The model under review builds one solid part; all positions refer to its coordinate system, in mm. A direction names the side the tool comes from. Coordinates: 2 decimals unless noted, no trailing zeros. Order: outer loops, then holes, each group sorted by start corner. A loop starts at its lowest first (then second) coordinate and runs counter-clockwise, first axis right, second up. Notation, with made-up numbers: M -33,-40 L -29,-40 A30 ccw -29,-13 Z; hole C 4,54.25 d5. An arc over 180 degrees is marked long. Write each question's results on one line, items separated by ' | '.
from build123d import *

# Parameters (mm, degrees)
F1_R     = 32.7
F1_R_2   = 5
F2_DEPTH = 1.8
F0_R     = 32.7
F3_DEPTH = 46.6
F4_R     = 2.65
F5_DEPTH = 44.601471
F6_R     = 5.5
F7_DEPTH = 39.6


with BuildPart() as f2:
    # F1 (on Front) → F2 (new body)
    with BuildSketch(Plane.XZ):
        Circle(F1_R)
        Circle(F1_R_2, mode=Mode.SUBTRACT)
    extrude(amount=F2_DEPTH)

    # F0 (on Front) → F3 (join)
    with BuildSketch(Plane.XZ):
        with BuildLine():
            ThreePointArc((32.077406, -10), (33.217171, -5.057625), (33.6, 0))
            ThreePointArc((33.6, 0), (33.217171, 5.057625), (32.077406, 10))
            ThreePointArc((32.077406, 10), (-33.6, 0), (32.077406, -10))
        make_face()
        Circle(F0_R, mode=Mode.SUBTRACT)
        with BuildLine():
            Line((42.851, 0), (33.6, 0))
            ThreePointArc((33.6, 0), (33.217171, -5.057625), (32.077406, -10))
            Line((32.077406, -10), (42.851, -10))
            Line((42.851, -10), (42.851, -4.75))
            Line((42.851, -4.75), (42.851, 0))
        make_face()
        with BuildLine():
            ThreePointArc((32.077406, 10), (33.217171, 5.057625), (33.6, 0))
            Line((33.6, 0), (42.851, 0))
            Line((42.851, 0), (42.851, 4.75))
            Line((42.851, 4.75), (42.851, 10))
            Line((42.851, 10), (32.077406, 10))
        make_face()
        Polygon((42.851, 4.75), (42.851, 0), (42.851, -4.75), (44.600471, -3), (44.600471, 3), align=None)
    extrude(amount=F3_DEPTH)

    # F4 (on Right) → F5 (cut, through all)
    with BuildSketch(Plane.YZ):
        with Locations((-11.8, 0)):
            Circle(F4_R)
        with Locations((-36.6, 0)):
            Circle(F4_R)
    extrude(amount=F5_DEPTH, mode=Mode.SUBTRACT)

    # F6 (on Right) → F7 (cut)
    with BuildSketch(Plane.YZ):
        with Locations((-11.8, 0)):
            Circle(F6_R)
        with Locations((-36.6, 0)):
            Circle(F6_R)
    extrude(amount=F7_DEPTH, mode=Mode.SUBTRACT)


solid = f2.part
1) For pin 1 (5 mm diameter, centred on y = -13, z = -7.5, fed in from -X); pin 2 (2 mm diameter, centred on x = 23, z = 11.5, fed in from -Y); pin 3 (8.5 mm diameter, centred on x = 38, y = -12.5, fed in from -Z); pin 4 (8 mm diameter, centred on x = 0, z = 0, fed in from -Y), all flat-tipped, find the tip position at first contact; note any pin that passes through.
Solutions:
pin 1: x = -33.23 | pin 2: y = -1.8 | pin 3: z = -10 | pin 4: through
2) Take a section at C-C on y = -22. State the section outline as (x, z) points, plus the area to 3 significant figures.
Solutions:
outline: M 32.08,-10 L 42.85,-10 L 42.85,-4.75 L 44.6,-3 L 44.6,3 L 42.85,4.75 L 42.85,10 L 32.08,10 A33.6 ccw long Z; hole C 0,0 d65.4 | area: 396 mm2
3) The part is to be moulded in two halves that separate along Z. For faces 6 (the cylindrical face through (-33.573, -22.974, 1.335)), 7 (the cylindrical face through (35.866, -17.295, 0.242)), 8 (the flat face through (37, -23, -10)), say which applies: pulls with the +Z half, pulls with the -Z half, needs draft (parallel to the pull), parting line crosses it, or undercut.
Solutions:
face 6: parting line crosses it | face 7: undercut | face 8: pulls with the -Z half
4) To check wall thickness, follow line 1 along Y through (x, z) = (42.8, 0); line 2 along Y through (x, z) = (35, 0); line 3 along Z through (x, y) = (0, -31). State the ranges of each line that lie inside material, in increasing order.
Solutions:
line 1: -46.6 to -39.25, -33.95 to -14.45, -9.15 to 0 | line 2: -46.6 to -42.1, -31.1 to -17.3, -6.3 to 0 | line 3: -33.6 to -32.7, 32.7 to 33.6
5) For faces 1 (the flat face through (7, -1.8, 0)), 2 (the cylindrical face through (42.065, -39.247, 0.117)), 3 (the flat face through (42.851, -23, -7)), 4 (the flat face through (42.851, -23, 7)), 5 (the flat face through (39.6, -35, 3)), list the 3-axis set-ups (+Z, -Z, +X, -X, +Y, -Y) from which the entire face can be reached by the end or side of a thin tool; tool diameter is ignored.
Solutions:
face 1: -Y | face 2: +X | face 3: -Z, +X, +Y, -Y | face 4: +Z, +X, +Y, -Y | face 5: none
6) Take a section at A-A on x = 0. State the section outline as (y, z) points, plus the area to 3 significant figures.
Solutions:
outline: M -46.6,-33.6 L 0,-33.6 L 0,-5 L -1.8,-5 L -1.8,-32.7 L -46.6,-32.7 Z; M -46.6,32.7 L -1.8,32.7 L -1.8,5 L 0,5 L 0,33.6 L -46.6,33.6 Z | area: 184 mm2
7) Take a section at B-B on z = 0. State the section outline as (x, y) points, plus the area to 3 significant figures.
Solutions:
outline: M -33.6,-46.6 L -32.7,-46.6 L -32.7,-1.8 L -5,-1.8 L -5,0 L -33.6,0 Z; M 5,-1.8 L 32.7,-1.8 L 32.7,-6.3 L 39.6,-6.3 L 39.6,-9.15 L 44.6,-9.15 L 44.6,0 L 5,0 Z; M 32.7,-46.6 L 44.6,-46.6 L 44.6,-39.25 L 39.6,-39.25 L 39.6,-42.1 L 32.7,-42.1 Z; M 32.7,-31.1 L 39.6,-31.1 L 39.6,-33.95 L 44.6,-33.95 L 44.6,-14.45 L 39.6,-14.45 L 39.6,-17.3 L 32.7,-17.3 Z | area: 491 mm2
8) Take a section at D-D on y = -36.6. State the section outline as (x, z) points, plus the area to 3 significant figures.
Solutions:
outline: M 32.08,-10 L 42.85,-10 L 42.85,-4.75 L 44.6,-3 L 44.6,-2.65 L 39.6,-2.65 L 39.6,-5.5 L 32.23,-5.5 A32.7 cw long 32.23,5.5 L 39.6,5.5 L 39.6,2.65 L 44.6,2.65 L 44.6,3 L 42.85,4.75 L 42.85,10 L 32.08,10 A33.6 ccw long Z | area: 292 mm2
